Design review of the part built by this model. Coordinates are the model's own, in mm. Face numbers are marked on the shaded views. Coordinates: 2 decimals unless noted, no trailing zeros. Loops run counter-clockwise (first coordinate to the right, second up) from the corner with the lowest first, then second, coordinate; pieces in that order, holes last. Notation, with made-up numbers: (54.5, 0.25) -> (70.5, 0.25) arc R16 ccw to (70.5, 12.25) -> close; hole circle Ø5 at (9, -20). An arc over 180 degrees is marked (long way). Answer in a Markdown table with one row per item.
```python
from build123d import *

# Parameters (mm, degrees)
ELBOW_HORN_FLANGE_PROFILE_R          = 13
ELBOW_HORN_FLANGE_DEPTH              = 4
FOREARM_WEB_PROFILE_W                = 40
FOREARM_WEB_PROFILE_H                = 14
FOREARM_WEB_DEPTH                    = 4
GRIPPER_MOUNT_RIB_PROFILE_W          = 8
GRIPPER_MOUNT_RIB_PROFILE_H          = 30
GRIPPER_MOUNT_RIB_DEPTH              = 4
GRIPPER_SERVO_MOUNT_PROFILE_W        = 44
GRIPPER_SERVO_MOUNT_PROFILE_H        = 26
GRIPPER_SERVO_MOUNT_DEPTH            = 4
GRIP_SG90_BODY_CLEARANCE_START       = -5
GRIP_SG90_BODY_CLEARANCE_PROFILE_W   = 23.8
GRIP_SG90_BODY_CLEARANCE_PROFILE_H   = 13
GRIP_SG90_BODY_CLEARANCE_DEPTH       = 87.221918224
MOVING_FINGER_SWEEP_RELIEF_START     = -5
MOVING_FINGER_SWEEP_RELIEF_PROFILE_W = 13
MOVING_FINGER_SWEEP_RELIEF_PROFILE_H = 13
MOVING_FINGER_SWEEP_RELIEF_DEPTH     = 87.221918224
GRIP_SERVO_TAB_FASTENERS_START       = -50
GRIP_SERVO_TAB_FASTENERS_PROFILE_R   = 1.3
GRIP_SERVO_TAB_FASTENERS_DEPTH       = 132.221918224
FIXED_FINGER_SPINE_PROFILE_W         = 48
FIXED_FINGER_SPINE_PROFILE_H         = 5
FIXED_FINGER_SPINE_DEPTH             = 4
FIXED_FINGER_ROOT_PROFILE_W          = 7
FIXED_FINGER_ROOT_PROFILE_H          = 23
FIXED_FINGER_ROOT_DEPTH              = 7
ELBOW_CENTER_SCREW_ACCESS_START      = -50
ELBOW_CENTER_SCREW_ACCESS_PROFILE_R  = 4
ELBOW_CENTER_SCREW_ACCESS_DEPTH      = 139.396832522
ELBOW_DOWEL_SUPPORT_HUB_START        = 4
ELBOW_DOWEL_SUPPORT_HUB_PROFILE_R    = 7
ELBOW_DOWEL_SUPPORT_HUB_PROFILE_R_2  = 4
ELBOW_DOWEL_SUPPORT_HUB_DEPTH        = 4
CAPTURED_HORN_KEY_BOSS_START         = -1.65
CAPTURED_HORN_KEY_BOSS_PROFILE_R     = 13
CAPTURED_HORN_KEY_BOSS_DEPTH         = 1.65
KEY_POCKET_HUB_START                 = -1.65
STOCK_HORN_POCKET_HUB_R              = 3.55
KEY_POCKET_HUB_DEPTH                 = 1.65
KEY_POCKET_HORIZONTAL_START          = -1.65
STOCK_HORN_POCKET_HORIZONTAL_W       = 16.3
STOCK_HORN_POCKET_HORIZONTAL_H       = 4.2
KEY_POCKET_HORIZONTAL_DEPTH          = 1.65
KEY_POCKET_VERTICAL_START            = -1.65
STOCK_HORN_POCKET_VERTICAL_W         = 4.2
STOCK_HORN_POCKET_VERTICAL_H         = 16.3
KEY_POCKET_VERTICAL_DEPTH            = 1.65
KEY_POCKET_ROUNDED_TIPS_START        = -1.65
STOCK_HORN_POCKET_ROUNDED_TIPS_R     = 2.1
KEY_POCKET_ROUNDED_TIPS_DEPTH        = 1.65
UNMODIFIED_HORN_CAPTURE_M2_START     = -50
UNMODIFIED_HORN_CAPTURE_M2_PROFILE_R = 1.15
UNMODIFIED_HORN_CAPTURE_M2_DEPTH     = 139.481636513
HUB_CLEARANCE_IN_KEY_BOSS_ONLY_START = -1.65
HORN_CENTER_HUB_CLEARANCE_R          = 4
HUB_CLEARANCE_IN_KEY_BOSS_ONLY_DEPTH = 1.65
FIXED_PAD_KEEPER_FASTENERS_START     = -50
FIXED_PAD_KEEPER_FASTENERS_PROFILE_R = 1.1
FIXED_PAD_KEEPER_FASTENERS_DEPTH     = 139.481636513


with BuildPart() as part:
    # Elbow_horn_flange_profile → Elbow_horn_flange (new body)
    with BuildSketch(Plane.XY):
        Circle(ELBOW_HORN_FLANGE_PROFILE_R)
    extrude(amount=ELBOW_HORN_FLANGE_DEPTH)

    # Forearm_web_profile → Forearm_web (add)
    with BuildSketch(Plane.XY):
        with Locations((20, 0)):
            Rectangle(FOREARM_WEB_PROFILE_W, FOREARM_WEB_PROFILE_H)
    extrude(amount=FOREARM_WEB_DEPTH)

    # Gripper_mount_rib_profile → Gripper_mount_rib (add)
    with BuildSketch(Plane.XY):
        with Locations((30, 15)):
            Rectangle(GRIPPER_MOUNT_RIB_PROFILE_W, GRIPPER_MOUNT_RIB_PROFILE_H)
    extrude(amount=GRIPPER_MOUNT_RIB_DEPTH)

    # Gripper_servo_mount_profile → Gripper_servo_mount (add)
    with BuildSketch(Plane.XY):
        with Locations((48, 28)):
            Rectangle(GRIPPER_SERVO_MOUNT_PROFILE_W, GRIPPER_SERVO_MOUNT_PROFILE_H)
    extrude(amount=GRIPPER_SERVO_MOUNT_DEPTH)

    # Grip_SG90_body_clearance_profile → Grip_SG90_body_clearance (cut, through all)
    with BuildSketch(Plane.XY.offset(GRIP_SG90_BODY_CLEARANCE_START)):
        with Locations((50.5, 30)):
            Rectangle(GRIP_SG90_BODY_CLEARANCE_PROFILE_W, GRIP_SG90_BODY_CLEARANCE_PROFILE_H)
    extrude(amount=GRIP_SG90_BODY_CLEARANCE_DEPTH, mode=Mode.SUBTRACT)

    # Moving_finger_sweep_relief_profile → Moving_finger_sweep_relief (cut, through all)
    with BuildSketch(Plane.XY.offset(MOVING_FINGER_SWEEP_RELIEF_START)):
        with Locations((64.5, 20.5)):
            Rectangle(MOVING_FINGER_SWEEP_RELIEF_PROFILE_W, MOVING_FINGER_SWEEP_RELIEF_PROFILE_H)
    extrude(amount=MOVING_FINGER_SWEEP_RELIEF_DEPTH, mode=Mode.SUBTRACT)

    # Grip_servo_tab_fasteners_profile → Grip_servo_tab_fasteners (cut, through all)
    with BuildSketch(Plane.XY.offset(GRIP_SERVO_TAB_FASTENERS_START)):
        with Locations((36, 30)):
            Circle(GRIP_SERVO_TAB_FASTENERS_PROFILE_R)
        with Locations((65, 30)):
            Circle(GRIP_SERVO_TAB_FASTENERS_PROFILE_R)
    extrude(amount=GRIP_SERVO_TAB_FASTENERS_DEPTH, mode=Mode.SUBTRACT)



with BuildPart() as body_2:
    # Fixed_finger_spine_profile → Fixed_finger_spine (new body)
    with BuildSketch(Plane.XY):
        with Locations((54, -13.5)):
            Rectangle(FIXED_FINGER_SPINE_PROFILE_W, FIXED_FINGER_SPINE_PROFILE_H)
    extrude(amount=FIXED_FINGER_SPINE_DEPTH)


with BuildPart() as part_1:
    add(part.part)

    add(body_2.part)  # Fixed_finger_root merges body 2
    # Fixed_finger_root_profile → Fixed_finger_root (add)
    with BuildSketch(Plane.XY):
        with Locations((30.5, -4.5)):
            Rectangle(FIXED_FINGER_ROOT_PROFILE_W, FIXED_FINGER_ROOT_PROFILE_H)
    extrude(amount=FIXED_FINGER_ROOT_DEPTH)

    # Elbow_center_screw_access_profile → Elbow_center_screw_access (cut, through all)
    with BuildSketch(Plane.XY.offset(ELBOW_CENTER_SCREW_ACCESS_START)):
        with Locations(Location((0, 0, 0), (0, 0, 180))):
            Circle(ELBOW_CENTER_SCREW_ACCESS_PROFILE_R)
    extrude(amount=ELBOW_CENTER_SCREW_ACCESS_DEPTH, mode=Mode.SUBTRACT)

    # Elbow_dowel_support_hub_profile → Elbow_dowel_support_hub (add)
    with BuildSketch(Plane.XY.offset(ELBOW_DOWEL_SUPPORT_HUB_START)):
        Circle(ELBOW_DOWEL_SUPPORT_HUB_PROFILE_R)
        with Locations(Location((0, 0, 0), (0, 0, 180))):
            Circle(ELBOW_DOWEL_SUPPORT_HUB_PROFILE_R_2, mode=Mode.SUBTRACT)
    extrude(amount=ELBOW_DOWEL_SUPPORT_HUB_DEPTH)

    # Captured_horn_key_boss_profile → Captured_horn_key_boss (add)
    with BuildSketch(Plane.XY.offset(CAPTURED_HORN_KEY_BOSS_START)):
        with Locations(Location((0, 0, 0), (0, 0, 32.578970393))):
            Circle(CAPTURED_HORN_KEY_BOSS_PROFILE_R)
    extrude(amount=CAPTURED_HORN_KEY_BOSS_DEPTH)

    # Stock_horn_pocket_Hub → Key_pocket_Hub (cut)
    with BuildSketch(Plane.XY.offset(KEY_POCKET_HUB_START)):
        Circle(STOCK_HORN_POCKET_HUB_R)
    extrude(amount=KEY_POCKET_HUB_DEPTH, mode=Mode.SUBTRACT)

    # Stock_horn_pocket_Horizontal → Key_pocket_Horizontal (cut)
    with BuildSketch(Plane.XY.offset(KEY_POCKET_HORIZONTAL_START)):
        Rectangle(STOCK_HORN_POCKET_HORIZONTAL_W, STOCK_HORN_POCKET_HORIZONTAL_H)
    extrude(amount=KEY_POCKET_HORIZONTAL_DEPTH, mode=Mode.SUBTRACT)

    # Stock_horn_pocket_Vertical → Key_pocket_Vertical (cut)
    with BuildSketch(Plane.XY.offset(KEY_POCKET_VERTICAL_START)):
        Rectangle(STOCK_HORN_POCKET_VERTICAL_W, STOCK_HORN_POCKET_VERTICAL_H)
    extrude(amount=KEY_POCKET_VERTICAL_DEPTH, mode=Mode.SUBTRACT)

    # Stock_horn_pocket_Rounded_tips → Key_pocket_Rounded_tips (cut)
    with BuildSketch(Plane.XY.offset(KEY_POCKET_ROUNDED_TIPS_START)):
        with Locations((8.15, 0)):
            Circle(STOCK_HORN_POCKET_ROUNDED_TIPS_R)
        with Locations((-8.15, 0)):
            Circle(STOCK_HORN_POCKET_ROUNDED_TIPS_R)
        with Locations((0, 8.15)):
            Circle(STOCK_HORN_POCKET_ROUNDED_TIPS_R)
        with Locations((0, -8.15)):
            Circle(STOCK_HORN_POCKET_ROUNDED_TIPS_R)
    extrude(amount=KEY_POCKET_ROUNDED_TIPS_DEPTH, mode=Mode.SUBTRACT)

    # Unmodified_horn_capture_M2_profile → Unmodified_horn_capture_M2 (cut, through all)
    with BuildSketch(Plane.XY.offset(UNMODIFIED_HORN_CAPTURE_M2_START)):
        with Locations(Location((7, 7, 0), (0, 0, 180))):
            Circle(UNMODIFIED_HORN_CAPTURE_M2_PROFILE_R)
        with Locations(Location((-7, 7, 0), (0, 0, 180))):
            Circle(UNMODIFIED_HORN_CAPTURE_M2_PROFILE_R)
        with Locations(Location((-7, -7, 0), (0, 0, 180))):
            Circle(UNMODIFIED_HORN_CAPTURE_M2_PROFILE_R)
        with Locations(Location((7, -7, 0), (0, 0, 180))):
            Circle(UNMODIFIED_HORN_CAPTURE_M2_PROFILE_R)
    extrude(amount=UNMODIFIED_HORN_CAPTURE_M2_DEPTH, mode=Mode.SUBTRACT)

    # Horn_center_hub_clearance → Hub_clearance_in_key_boss_only (cut)
    with BuildSketch(Plane.XY.offset(HUB_CLEARANCE_IN_KEY_BOSS_ONLY_START)):
        with Locations(Location((0, 0, 0), (0, 0, 148.331756746))):
            Circle(HORN_CENTER_HUB_CLEARANCE_R)
    extrude(amount=HUB_CLEARANCE_IN_KEY_BOSS_ONLY_DEPTH, mode=Mode.SUBTRACT)

    # Fixed_pad_keeper_fasteners_profile → Fixed_pad_keeper_fasteners (cut, through all)
    with BuildSketch(Plane.XY.offset(FIXED_PAD_KEEPER_FASTENERS_START)):
        with Locations(Location((57, -13.5, 0), (0, 0, 180))):
            Circle(FIXED_PAD_KEEPER_FASTENERS_PROFILE_R)
        with Locations(Location((73, -13.5, 0), (0, 0, 180))):
            Circle(FIXED_PAD_KEEPER_FASTENERS_PROFILE_R)
    extrude(amount=FIXED_PAD_KEEPER_FASTENERS_DEPTH, mode=Mode.SUBTRACT)


solid = part_1.part
```
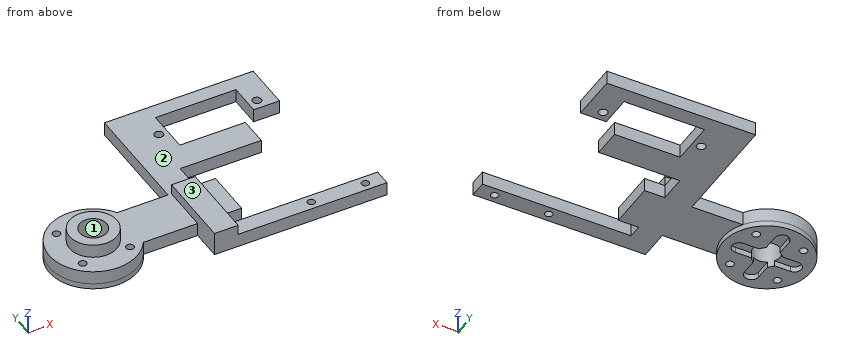
(1) Draft analysis for pull direction X (two halves, no side actions). For the marked faces 1, 2 and 3, state which applies: pulls with the +X half, pulls with the -X half, needs draft (parallel to the pull), parting line crosses it, or undercut.
Evaluation:
| item | result |
|---|---|
| face 1 | undercut |
| face 2 | undercut |
| face 3 | needs draft |
(2) For pin 1 (2 mm diameter, centred on x = 28, y = 19, fed in from +Z); pin 2 (10 mm diameter, centred on x = 29, y = 5.5, fed in from +Z); pin 3 (2 mm diameter, centred on y = 37, z = 2.5, fed in from +X), all flat-tipped, find the tip position at first contact; note any pin that passes through.
Evaluation:
| item | result |
|---|---|
| pin 1 | stops at z = 4 |
| pin 2 | stops at z = 7 |
| pin 3 | stops at x = 70 |
(3) Take a section at B-B on x = 57. Give the boundary of the cut face in (y, z), and give its area (3 significant figures).
Evaluation:
| item | result |
|---|---|
| outline | (-16, 0) -> (-14.6, 0) -> (-14.6, 4) -> (-16, 4) -> close; (-12.4, 0) -> (-11, 0) -> (-11, 4) -> (-12.4, 4) -> close; (15, 0) -> (23.5, 0) -> (23.5, 4) -> (15, 4) -> close; (36.5, 0) -> (41, 0) -> (41, 4) -> (36.5, 4) -> close |
| area | 63.2 mm² |
(4) Take a section at C-C on z = 2. Count the separate pieces of the cut face and the enclosed holes in it, and give its area (3 significant figures).
Evaluation:
| item | result |
|---|---|
| separate pieces | 1 |
| enclosed holes | 9 |
| area | 1,890 mm² |
(5) Take a section at A-A on y = 35. Give the boundary of the cut face in (x, z), and give its area (3 significant figures).
Evaluation:
| item | result |
|---|---|
| outline | (26, 0) -> (38.6, 0) -> (38.6, 4) -> (26, 4) -> close; (62.4, 0) -> (70, 0) -> (70, 4) -> (62.4, 4) -> close |
| area | 80.8 mm² |
(6) To check wall thickness, follow probe 1 along Y at (x, z) = (36, 1.5); probe 2 along Y at (x, z) = (57, 1.6); probe 3 along Y at (x, z) = (55.5, 3.75). State the ranges of each line that lie inside material, in increasing order.
Evaluation:
| item | result |
|---|---|
| probe 1 | y = -16 to -11, -7 to 7, 15 to 28.7, 31.3 to 41 |
| probe 2 | y = -16 to -14.6, -12.4 to -11, 15 to 23.5, 36.5 to 41 |
| probe 3 | y = -16 to -11, 15 to 23.5, 36.5 to 41 |
(7) Take a section at D-D on x = 0. Give the boundary of the cut face in (y, z), and give its area (3 significant figures).
Evaluation:
| item | result |
|---|---|
| outline | (-13, -1.65) -> (-10.25, -1.65) -> (-10.25, 0) -> (-4, 0) -> (-4, 8) -> (-7, 8) -> (-7, 4) -> (-13, 4) -> close; (4, 0) -> (10.25, 0) -> (10.25, -1.65) -> (13, -1.65) -> (13, 4) -> (7, 4) -> (7, 8) -> (4, 8) -> close |
| area | 105 mm² |
